Read the model definition and answer for the solid it produces. Units are mm, in the model's axes. A direction names the side the tool comes from. Give positions to 0.01 mm unless a question says otherwise; leave off trailing zeros. Loops run counter-clockwise (first coordinate to the right, second up) from the corner with the lowest first, then second, coordinate; pieces in that order, holes last. Notation, with made-up numbers: (32, 17.25) - (43, 17.25) arc R25 cw to (43, 30.25) - close; hole circle Ø7 at (56, 65.5). An arc over 180 degrees is marked (long way). Write each question's results on one line, items separated by ' | '. Start each with the question number.
Q1. The part is cut by section D-D, the plane x = -23.5. Write down the section's boundary in (y, z).
Q2. The part is cut by section A-A, the plane y = 6.5. Write down the section's boundary in (x, z), plus the area to 3 significant figures.
Q3. Find the intervals of material crossed by line 1 (Z direction, x = 15, y = 6.9); line 2 (X direction, y = 4.85, z = 5); line 3 (Z direction, x = 1, y = 2.75), in increasing order. Write a range as from..to.
Q4. For faces 1 (the cylindrical face through (-16.126, 5.465, -21.228)), 2 (the flat face through (16, 8, -1)), determine the directions among +Z, -Z, +X, -X, +Y, -Y from which every point of the face is accessible in a straight line to the end or side of a thin tool.
Q5. The part is cut by section B-B, the plane x = 0. Write down the section's boundary in (y, z).
Q6. The part is cut by section C-C, the plane z = -1. Write down the section's boundary in (x, y), plus the area to 3 significant figures.
Q7. Given pin 1 (2 mm diameter, centred on y = 3, z = 8.5, fed in from +X); pin 2 (4 mm diameter, centred on x = 2, y = 5, fed in from -Z); pin 3 (4 mm diameter, centred on x = -1.5, y = 6, fed in from +Z), each flat-ended and moving along its own axis, determine where each tip first touches the part or whether it passes through.
Q8. Determine the mould class of faces 3 (the flat face through (-1, 0, -1)), 4 (the cylindrical face through (17.535, 3.944, -33.713)), 5 (the flat face through (10, 4, 0)) for opening direction X: +X half, -X half, draft (parallel to the pull), parting line (faces both ways), or undercut.
Autodesk Fusion 360 part; units mm, degrees
sketch "Sketch1" plane through (0, 0, 0) normal (0, 1, 0) x (1, 0, 0)
  circle A0 centre (0, 0) radius 38
  line L0 (-10, 25) -> (10, 25)
  line L1 (10, 25) -> (10, -25)
  line L2 (10, -25) -> (-10, -25)
  line L3 (-10, -25) -> (-10, 25)
  line L4 (1.75, 0) -> (22.5, 0) construction
  line L5 (0, -1.75) -> (0, -22.5) construction
  dimension "d1" = 76
  dimension "d2" = 20
  dimension "d3" = 50
extrude "Extrude1" add sketch "Sketch1" along normal blind 8
extrude "Extrude2" add sketch "Sketch1" along normal blind 0.5 contours L0 L1 L2 L3
sketch "Sketch2" plane through (0, 8, 0) normal (0, 1, 0) x (-1, 0, 0)
  line L0 (-10, 25) -> (10, 25)
  line L1 (10, 25) -> (10, -25)
  line L2 (10, -25) -> (-10, -25)
  line L3 (-10, -25) -> (-10, 25)
  circle A0 centre (0, 0) radius 38
  line L4 (0, 1.75) -> (0, 22.5)
  line L5 (-1.75, 0) -> (-22.5, 0)
  point P0 (15, -20)
  point P1 (15, 5)
  point P2 (-15, -20)
  point P3 (-15, 5)
  dimension "d10" = 30
  dimension "d11" = 25
  dimension "d12" = 20
hole "Hole1" at (-15, 8, -20) at (-15, 8, 5) at (15, 8, -20) at (15, 8, 5) direction (0, -1, 0) diameter 3.332 depth 5 tip angle 118
fillet "Fillet1" radius 5 4 edges at (-10, 4.25, 25) (-10, 4.25, -25) (10, 4.25, 25) (10, 4.25, -25)
equation "d1 = ( 38 * 2 ) * 1 mm"
Check sheet entries:
1) outline: (0, -29.86) - (8, -29.86) - (8, 29.86) - (0, 29.86) - close
2) outline: circle Ø76 at (0, 0); hole circle Ø3.33 at (-15, -20); hole circle Ø3.33 at (-15, 5); hole (-10, -20) arc R5 ccw to (-5, -25) - (5, -25) arc R5 ccw to (10, -20) - (10, 20) arc R5 ccw to (5, 25) - (-5, 25) arc R5 ccw to (-10, 20) - close; hole circle Ø3.33 at (15, -20); hole circle Ø3.33 at (15, 5) | area: 3,520 mm^2
3) line 1: z = -34.91..-21.67, -18.33..3.33, 6.67..34.91 | line 2: x = -37.67..-16.67, -13.33..-10, 10..13.33, 16.67..37.67 | line 3: z = -37.99..-25, 25..37.99
4) face 1: +Y | face 2: +Z, -Z, +X, -X, +Y
5) outline: (0, -38) - (8, -38) - (8, -25) - (0.5, -25) - (0.5, 25) - (8, 25) - (8, 38) - (0, 38) - close
6) outline: (-37.99, 0) - (37.99, 0) - (37.99, 8) - (10, 8) - (10, 0.5) - (-10, 0.5) - (-10, 8) - (-37.99, 8) - close | area: 458 mm^2
7) pin 1: stops at x = 37.25 | pin 2: stops at z = -38 | pin 3: stops at z = 38
8) face 3: draft | face 4: parting line | face 5: undercut
